from build123d import *

# Parameters (mm, degrees)
F0_W     = 77.0167037845
F0_H     = 19.9013762176
F1_DEPTH = 63.5
F2_W     = 31.3891619444
F2_H     = 64.5581185818
F3_DEPTH = 127
F4_SIZE2 = 5.08
F4_SIZE  = 5.08


# Not quite as in the source:
# - the program builds the solid bodies; features that only make, move or delete a surface that nothing else refers to are left out


with BuildPart() as f1:
    # F0 (on Front) → F1 (new body, symmetric)
    with BuildSketch(Plane.XZ):
        Rectangle(F0_W, F0_H)
    extrude(amount=F1_DEPTH, both=True)

    # F2 (on Top) → F3 (join)
    with BuildSketch(Plane.XY):
        Rectangle(F2_W, F2_H)
    extrude(amount=F3_DEPTH)

    # F4
    f4_edges = [f1.edges().sort_by_distance(p)[0] for p in [
        (0, -32.279059, 127),
        (15.694581, -32.279059, 68.475344),
        (0, 32.279059, 127),
        (15.694581, 0, 127),
        (-15.694581, 0, 127),
        (15.694581, 32.279059, 68.475344),
        (-15.694581, 32.279059, 68.475344),
        (-15.694581, -32.279059, 68.475344),
        (15.694581, 0, 9.950688),
        (38.508352, 0, 9.950688),
        (0, -63.5, 9.950688),
        (0, 63.5, 9.950688),
        (-38.508352, 0, 9.950688),
        (0, -63.5, -9.950688),
        (-38.508352, 0, -9.950688),
        (0, 63.5, -9.950688),
        (38.508352, 0, -9.950688),
        (38.508352, 63.5, 0),
        (-38.508352, 63.5, 0),
        (38.508352, -63.5, 0),
        (-38.508352, -63.5, 0),
        (-15.694581, 0, 9.950688),
        (0, -32.279059, 9.950688),
        (0, 32.279059, 9.950688),
    ]]
    chamfer(f4_edges, length=F4_SIZE, length2=F4_SIZE2)


solid = f1.part
The listing builds one solid part. Answer for the finished solid, in the listing's coordinates (mm). A direction names the side the tool comes from. Coordinates: 2 decimals unless noted, no trailing zeros. Write each loop counter-clockwise with the first axis right and the second up, starting at its lowest first coordinate (ties: lowest second). Pieces come first, ordered by that corner, then holes. Notation, with made-up numbers: (44, 50.5) - (80, 50.5) arc R5 ccw to (80, 56.5) - close; hole circle Ø2 at (-26.5, 21). An arc over 180 degrees is marked (long way). Return JSON: item names as keys, results as strings.
1. The part is cut by section C-C on z = 18. Determine the outline of the cut face in (x, y).
Final values:
{"outline": "(-15.69, -27.2) - (-10.61, -32.28) - (10.61, -32.28) - (15.69, -27.2) - (15.69, 27.2) - (10.61, 32.28) - (-10.61, 32.28) - (-15.69, 27.2) - close"}
2. Consider line 1 along Y through (x, z) = (-8, 18.5); line 2 along X through (y, z) = (-22, 89.5); line 3 along Z through (x, y) = (-21.5, 9). Determine where each line is inside the solid, lowest interval first.
Final values:
{"line 1": "-32.28 to 32.28", "line 2": "-15.69 to 15.69", "line 3": "-9.95 to 9.95"}
3. The part is cut by section A-A on x = -31. Determine the outline of the cut face in (y, z).
Final values:
{"outline": "(-63.5, -4.87) - (-58.42, -9.95) - (58.42, -9.95) - (63.5, -4.87) - (63.5, 4.87) - (58.42, 9.95) - (-58.42, 9.95) - (-63.5, 4.87) - close"}
4. The part is cut by section B-B on y = 13.5. Determine the outline of the cut face in (x, z), then the cut area to 3 significant figures.
Final values:
{"outline": "(-38.51, -4.87) - (-33.43, -9.95) - (33.43, -9.95) - (38.51, -4.87) - (38.51, 4.87) - (33.43, 9.95) - (20.77, 9.95) - (15.69, 15.03) - (15.69, 121.92) - (10.61, 127) - (-10.61, 127) - (-15.69, 121.92) - (-15.69, 15.03) - (-20.77, 9.95) - (-33.43, 9.95) - (-38.51, 4.87) - close", "area": "5,160 mm^2"}
5. The part is cut by section D-D on x = 2.5. Determine the outline of the cut face in (y, z), then the cut area to 3 significant figures.
Final values:
{"outline": "(-63.5, -4.87) - (-58.42, -9.95) - (58.42, -9.95) - (63.5, -4.87) - (63.5, 4.87) - (58.42, 9.95) - (37.36, 9.95) - (32.28, 15.03) - (32.28, 121.92) - (27.2, 127) - (-27.2, 127) - (-32.28, 121.92) - (-32.28, 15.03) - (-37.36, 9.95) - (-58.42, 9.95) - (-63.5, 4.87) - close", "area": "10,000 mm^2"}
6. Each of these flat-tipped pins is pushed along its axis until it touches: pin 1 Ø23.5 at (x, z) = (1, 74.5) entering from -Y; pin 2 Ø3 at (y, z) = (0, 52) entering from +X; pin 3 Ø1.5 at (x, z) = (-10.5, 101) entering from +Y. Where does it stop, or does it pass through?
Final values:
{"pin 1": "y = -32.28", "pin 2": "x = 15.69", "pin 3": "y = 32.28"}
7. Which of the six approach directions +Z, -Z, +X, -X, +Y, -Y give full straight-line access (tool end or side, diameter ignored) to faces 1 (the face through (-13.119, 29.775, 67.727)), 2 (the face through (0, 32.279, 68)), 3 (the face through (13.19, -29.703, 67.727))?
Final values:
{"face 1": "+Z, -X, +Y", "face 2": "+Z, +X, -X, +Y", "face 3": "+Z, +X, -Y"}
